Part model, mm, in its own coordinate system. Round coordinates to 2 decimals unless told otherwise and drop trailing zeros. Write each loop counter-clockwise with the first axis right and the second up, starting at its lowest first coordinate (ties: lowest second). Pieces come first, ordered by that corner, then holes. Notation, with made-up numbers: (-0.75, 89) -> (58.25, 89) arc R25 ccw to (58.25, 128) -> close; hole circle Ø4 at (8.5, 86.5). An arc over 180 degrees is marked (long way). Return JSON: item names as keys, results as strings. Group by question number.
```python
from build123d import *

# Parameters (mm, degrees)
F0_R     = 100
F1_DEPTH = 3
F3_D     = 10
F4_D     = 5


with BuildPart() as f1:
    # F0 (on Top) → F1 (new body)
    with BuildSketch(Plane.XY):
        Circle(F0_R)
    extrude(amount=F1_DEPTH)

    # F3 (through all)
    with Locations(Plane.XY.offset(3)):
        with Locations((0, 0)):
            Hole(F3_D / 2)

    # F4 (through all)
    with Locations(Plane.XY.offset(3)):
        with Locations((-10, -95), (10, -95), (87.272413, 38.839746), (77.272413, 56.160254), (-77.272413, 56.160254), (-87.272413, 38.839746)):
            Hole(F4_D / 2)


solid = f1.part
```
Item 1: Cut at D-D (x = 28). Write the cut outline in (y, z).
Item 2: Cut at A-A (x = 0). Write the cut outline in (y, z), then the cut area to 3 significant figures.
Item 3: Flat gauge pins, fed straight in: P1, Ø1.5, axis at y = 4.5, z = 2, coming from the +X side; P2, Ø3, axis at x = -87.27, y = 38.84, coming from the -Z side. Where does each tip first touch, or does it go through?
Item 4: Two-plate mould, pull along Y, no slides. Class faces 1 (the face through (-75.43, 57.85, 1.48)), 2 (the face through (-1, -21, 3)), 3 (the face through (95.38, 30.04, 1.48)), 4 (the face through (-85.43, 40.53, 1.48)): released by +Y, released by -Y, zero draft, split by the parting line, or undercut.
Item 5: Cut at C-C (z = 1.75). Write the cut outline in (x, y), then the cut area to 3 significant figures.
Item 6: Wall check: L1, parallel to Y at x = 0, z = 1.95; L2, parallel to Y at x = -10, z = 1.4; L3, parallel to Y at x = -33.5, z = 1.75. Give the ranges that are in metal, low to high.
Checks:
{
 "1": {"outline": "(-96, 0) -> (96, 0) -> (96, 3) -> (-96, 3) -> close"},
 "2": {"outline": "(-100, 0) -> (-5, 0) -> (-5, 3) -> (-100, 3) -> close; (5, 0) -> (100, 0) -> (100, 3) -> (5, 3) -> close", "area": "570 mm2"},
 "3": {"P1": "stops at x = 99.93", "P2": "passes through"},
 "4": {"face 1": "undercut", "face 2": "zero draft", "face 3": "split by the parting line", "face 4": "undercut"},
 "5": {"outline": "circle Ø200 at (0, 0); hole circle Ø5 at (-87.27, 38.84); hole circle Ø5 at (-77.27, 56.16); hole circle Ø5 at (-10, -95); hole circle Ø10 at (0, 0); hole circle Ø5 at (10, -95); hole circle Ø5 at (77.27, 56.16); hole circle Ø5 at (87.27, 38.84)", "area": "31,200 mm2"},
 "6": {"L1": "y = -100 to -5, 5 to 100", "L2": "y = -99.5 to -97.5, -92.5 to 99.5", "L3": "y = -94.22 to 94.22"}
}
